Job drawing, mm, ordinate dimensions from the low corner. One solid piece. Give positions to 0.01 mm unless a question says otherwise; leave off trailing zeros. Order: outer loops, then holes, each group sorted by start corner. A loop starts at its lowest first (then second) coordinate and runs counter-clockwise, first axis right, second up.
1. Drop flat-ended pins along their axis: pin 1 Ø4 at (y, z) = (30, 55.5) entering from -X; pin 2 Ø1.2 at (x, y) = (1, 35) entering from +Z; pin 3 Ø2 at (x, z) = (3, 72) entering from +Y; pin 4 Ø9 at (y, z) = (18, 18) entering from -X. Give the stop position or say it passes through.
2. Probe line 1 (Y direction, x = 3.1, z = 54); line 2 (Z direction, x = 1.75, y = 20); line 3 (Y direction, x = 2.8, z = 36). List the from-to ranges inside material, lowest first.
3. Slice it at D-D on z = 36. List the corners of the cut face in (x, y).
4. Slice it at C-C on x = 3.4. List the corners of the cut face in (y, z), and give its area (3 significant figures).
5. Slice it at A-A on z = 54. List the corners of the cut face in (x, y), and give its area (3 significant figures).
6. Slice it at B-B on y = 19. List the corners of the cut face in (x, z), and give its area (3 significant figures).
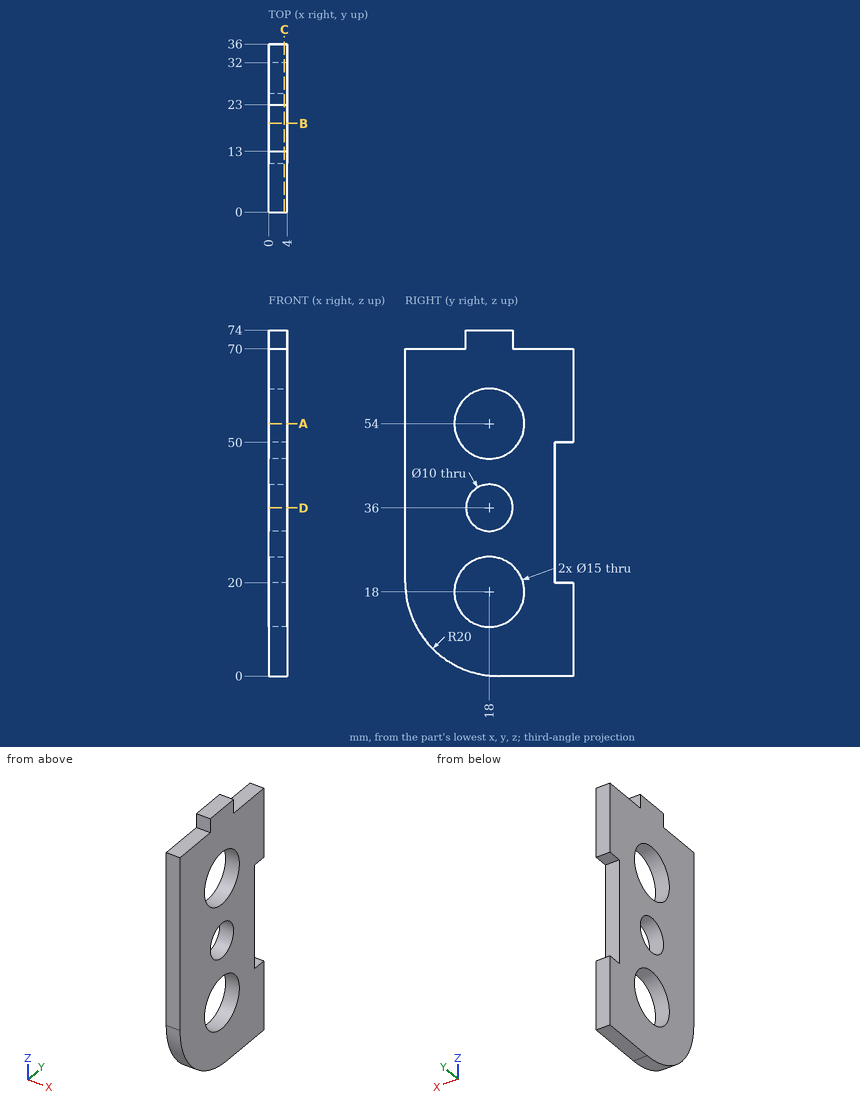
Data:
1. pin 1: stops at x = 0
1. pin 2: stops at z = 70
1. pin 3: stops at y = 23
1. pin 4: passes through
2. line 1: y = 0 to 10.5, 25.5 to 36
2. line 2: z = 0 to 10.77, 25.23 to 31.42, 40.58 to 46.77, 61.23 to 74
2. line 3: y = 0 to 13, 23 to 32
3. outline: (0, 0) - (4, 0) - (4, 13) - (0, 13) - close; (0, 23) - (4, 23) - (4, 32) - (0, 32) - close
4. outline: (0, 20) arc R20 ccw to (20, 0) - (36, 0) - (36, 20) - (32, 20) - (32, 50) - (36, 50) - (36, 70) - (23, 70) - (23, 74) - (13, 74) - (13, 70) - (0, 70) - close; hole circle Ø15 at (18, 18); hole circle Ø15 at (18, 54); hole circle Ø10 at (18, 36)
4. area: 1,920 mm2
5. outline: (0, 0) - (4, 0) - (4, 10.5) - (0, 10.5) - close; (0, 25.5) - (4, 25.5) - (4, 36) - (0, 36) - close
5. area: 84.0 mm2
6. outline: (0, 0.03) - (4, 0.03) - (4, 10.57) - (0, 10.57) - close; (0, 25.43) - (4, 25.43) - (4, 31.1) - (0, 31.1) - close; (0, 40.9) - (4, 40.9) - (4, 46.57) - (0, 46.57) - close; (0, 61.43) - (4, 61.43) - (4, 74) - (0, 74) - close
6. area: 138 mm2
